from build123d import *

# Parameters (mm, degrees)
BOSS_EXTRUDE1_DEPTH = 23.0378
SKETCH2_R           = 3.683
BOSS_EXTRUDE2_DEPTH = 1.7272
SKETCH3_R           = 1.7526
CUT_EXTRUDE1_DEPTH  = 58.8104
BOSS_EXTRUDE3_DEPTH = 2.032


with BuildPart() as part:
    # Sketch1 → Boss-Extrude1 (new body)
    with BuildSketch(Plane(origin=(0, 0, 0), x_dir=(1, 0, 0), z_dir=(0, 1, 0))):
        Polygon((-34.798, 19.2532), (-24.384, 19.2532), (-24.384, 17.399), (-4.3942, 17.399), (-4.3942, 23.684705806), (2.0701, 23.684705806), (2.0701, 27.178), (28.3337, 27.178), (28.3337, 23.6728), (34.798, 23.6728), (34.798, -23.6728), (28.3337, -23.6728), (28.3337, -27.178), (2.0701, -27.178), (2.0701, -23.684705806), (-4.3942, -23.684705806), (-4.3942, -17.399), (-24.384, -17.399), (-24.384, -19.2532), (-34.798, -19.2532), align=None)
    extrude(amount=BOSS_EXTRUDE1_DEPTH)

    # Sketch2 → Boss-Extrude2 (add)
    with BuildSketch(Plane.XY.offset(27.178)):
        with Locations((21.1963, 11.5189)):
            Circle(SKETCH2_R)
        with Locations((9.2075, 11.5189)):
            Circle(SKETCH2_R)
    boss_extrude2 = extrude(amount=BOSS_EXTRUDE2_DEPTH)

    # Mirror1: Boss-Extrude2 across plane
    add(boss_extrude2.mirror(Plane.XY))

    # Sketch3 → Cut-Extrude1 (cut, through all)
    with BuildSketch(Plane.XY.offset(28.9052)):
        with Locations((21.1963, 11.5189)):
            Circle(SKETCH3_R)
        with Locations((9.2075, 11.5189)):
            Circle(SKETCH3_R)
    extrude(amount=-CUT_EXTRUDE1_DEPTH, mode=Mode.SUBTRACT)

    # Sketch4 → Boss-Extrude3 (add)
    with BuildSketch(Plane(origin=(0, 23.0378, 0), x_dir=(1, 0, 0), z_dir=(0, 1, 0))):
        with BuildLine():
            Line((13.5509, -27.178), (9.652, -27.178))
            Line((9.652, -27.178), (12.067809158, -32.389905736))
            ThreePointArc((12.067809158, -32.389905736), (15.2019, -34.3916), (18.335990842, -32.389905736))
            Line((18.335990842, -32.389905736), (20.7518, -27.178))
            Line((20.7518, -27.178), (16.8529, -27.178))
            Line((16.8529, -27.178), (16.8529, -30.9372))
            ThreePointArc((16.8529, -30.9372), (15.2019, -32.5882), (13.5509, -30.9372))
            Line((13.5509, -30.9372), (13.5509, -27.178))
        make_face()
        with BuildLine():
            Line((16.8529, 30.9372), (16.8529, 27.178))
            Line((16.8529, 27.178), (20.7518, 27.178))
            Line((20.7518, 27.178), (18.335990842, 32.389905736))
            ThreePointArc((18.335990842, 32.389905736), (15.2019, 34.3916), (12.067809158, 32.389905736))
            Line((12.067809158, 32.389905736), (9.652, 27.178))
            Line((9.652, 27.178), (13.5509, 27.178))
            Line((13.5509, 27.178), (13.5509, 30.9372))
            ThreePointArc((13.5509, 30.9372), (15.2019, 32.5882), (16.8529, 30.9372))
        make_face()
    extrude(amount=-BOSS_EXTRUDE3_DEPTH)


solid = part.part
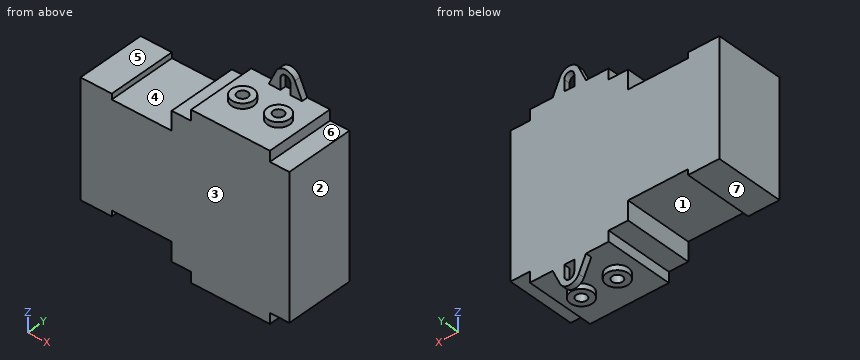
Work out the finished part from the listing and answer in its coordinate system (mm). Face numbers are marked on the shaded views. A direction names the side the tool comes from. Give positions to 0.01 mm unless a question says otherwise; leave off trailing zeros. Loops run counter-clockwise (first coordinate to the right, second up) from the corner with the lowest first, then second, coordinate; pieces in that order, holes last. Notation, with made-up numbers: (45, 64.25) -> (69, 64.25) arc R22 ccw to (69, 80.25) -> close; hole circle Ø6 at (-10, -21.75). An arc over 180 degrees is marked (long way). Use a Markdown table: item, result. Add a question column.
1. Section B-B on x = -14 is taken. Determine the outline of the cut face in (y, z), and give its area (3 significant figures).
2. Flat-ended cylindrical pins translate along their axes: pin 1 Ø12 at (x, y) = (22, 3.5) entering from +Z; pin 2 Ø0.6 at (y, z) = (22.5, 29) entering from -X; pin 3 Ø8 at (x, y) = (-11.5, 7.5) entering from +Z; pin 4 Ø7 at (y, z) = (16.5, 20.5) entering from -X. Find the tip coordinate at first contact, or state that the pin passes through.
3. Section C-C on z = 21 is taken. Determine the outline of the cut face in (x, y), and give its area (3 significant figures).
4. Section D-D on x = -26.5 is taken. Determine the outline of the cut face in (y, z).
5. Section A-A on y = 17.5 is taken. Determine the outline of the cut face in (x, z).
6. Find the intervals of material crossed by probe 1 along X at (y, z) = (13, -26.5); probe 2 along Z at (x, y) = (0, 3.75); probe 3 along X at (y, z) = (15.5, -20), in increasing order.
7. Determine the mould class of the marked faces 1, 2 and 3 for opening direction X: released by +X, released by -X, zero draft, split by the parting line, or undercut.
8. For the marked faces 4, 5, 6 and 7, determine the directions among +Z, -Z, +X, -X, +Y, -Y from which every point of the face is accessible in a straight line to the end or side of a thin tool.
Results below:
| question | item | result |
|---|---|---|
| 1 | outline | (0, -17.4) -> (23.04, -17.4) -> (23.04, 17.4) -> (0, 17.4) -> close |
| 1 | area | 802 mm^2 |
| 2 | pin 1 | stops at z = 28.91 |
| 2 | pin 2 | stops at x = 10.36 |
| 2 | pin 3 | stops at z = 17.4 |
| 2 | pin 4 | stops at x = -34.8 |
| 3 | outline | (-4.39, 0) -> (34.8, 0) -> (34.8, 23.04) -> (-4.39, 23.04) -> close; hole circle Ø3.51 at (9.21, 11.52); hole circle Ø3.51 at (21.2, 11.52) |
| 3 | area | 884 mm^2 |
| 4 | outline | (0, -19.25) -> (23.04, -19.25) -> (23.04, 19.25) -> (0, 19.25) -> close |
| 5 | outline | (-34.8, -19.25) -> (-24.38, -19.25) -> (-24.38, -17.4) -> (-4.39, -17.4) -> (-4.39, -23.68) -> (2.07, -23.68) -> (2.07, -27.18) -> (28.33, -27.18) -> (28.33, -23.67) -> (34.8, -23.67) -> (34.8, 23.67) -> (28.33, 23.67) -> (28.33, 27.18) -> (2.07, 27.18) -> (2.07, 23.68) -> (-4.39, 23.68) -> (-4.39, 17.4) -> (-24.38, 17.4) -> (-24.38, 19.25) -> (-34.8, 19.25) -> close |
| 6 | probe 1 | x = 2.07 to 8.27, 10.14 to 20.26, 22.13 to 28.33 |
| 6 | probe 2 | z = -23.68 to 23.68 |
| 6 | probe 3 | x = -4.39 to 34.8 |
| 7 | face 1 | undercut |
| 7 | face 2 | released by +X |
| 7 | face 3 | zero draft |
| 8 | face 4 | +Z, +Y, -Y |
| 8 | face 5 | +Z, -X, +Y, -Y |
| 8 | face 6 | +Z, +X, +Y, -Y |
| 8 | face 7 | -Z, -X, +Y, -Y |
